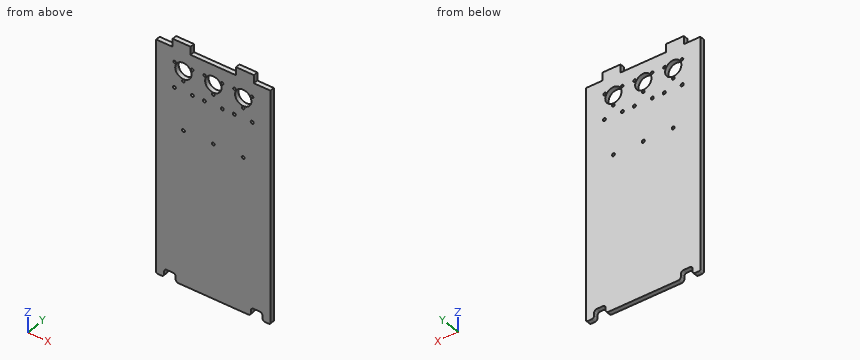
Autodesk Inventor part; units mm, degrees
ref_plane "YZ Plane" through (0, 0, 0) normal (1, 0, 0) x (0, 1, 0)
ref_plane "XZ Plane" through (0, 0, 0) normal (0, 1, 0) x (-1, 0, 0)
ref_plane "XY Plane" through (0, 0, 0) normal (0, 0, 1) x (1, 0, 0)
sketch "Sketch1" plane through (0, 0, 0) normal (0, 1, 0) x (-1, 0, 0)
  line L0 (-41.5, -207.85) -> (-41.5, -204.85)
  line L1 (-44.5, -201.85) -> (-51.2, -201.85)
  line L2 (-54.2, -204.85) -> (-54.2, -207.85)
  line L3 (-57.2, -210.85) -> (-61.5, -210.85)
  arc A0 (-41.5, -207.85) -> (-38.5, -210.85) centre (-38.5, -207.85) ccw
  arc A1 (-41.5, -204.85) -> (-44.5, -201.85) centre (-44.5, -204.85) ccw
  arc A2 (-51.2, -201.85) -> (-54.2, -204.85) centre (-51.2, -204.85) ccw
  arc A3 (-57.2, -210.85) -> (-54.2, -207.85) centre (-57.2, -207.85) ccw
  line L4 (41.5, -207.85) -> (41.5, -204.85)
  line L5 (44.5, -201.85) -> (51.2, -201.85)
  line L6 (54.2, -204.85) -> (54.2, -207.85)
  line L7 (61.5, -210.85) -> (57.2, -210.85)
  line L8 (38.5, -210.85) -> (-38.5, -210.85)
  arc A4 (54.2, -207.85) -> (57.2, -210.85) centre (57.2, -207.85) ccw
  arc A5 (54.2, -204.85) -> (51.2, -201.85) centre (51.2, -204.85) ccw
  arc A6 (44.5, -201.85) -> (41.5, -204.85) centre (44.5, -204.85) ccw
  arc A7 (38.5, -210.85) -> (41.5, -207.85) centre (38.5, -207.85) ccw
  line L9 (44.75, 48.15) -> (25.05, 48.15)
  line L10 (25.05, 48.15) -> (25.05, 57.15)
  line L11 (25.05, 57.15) -> (44.75, 57.15)
  line L12 (44.75, 57.15) -> (44.75, 48.15)
  line L13 (-25.05, 48.15) -> (-44.75, 48.15)
  line L14 (-44.75, 48.15) -> (-44.75, 57.15)
  line L15 (-44.75, 57.15) -> (-25.05, 57.15)
  line L16 (-25.05, 57.15) -> (-25.05, 48.15)
  line L17 (44.75, 48.15) -> (63, 48.15)
  line L18 (25.05, 48.15) -> (-25.05, 48.15)
  line L19 (-44.75, 48.15) -> (-63, 48.15)
  line L20 (63, -209.35) -> (63, 48.15)
  line L21 (-63, -209.35) -> (-63, 48.15)
  arc A8 (61.5, -210.85) -> (63, -209.35) centre (61.5, -209.35) ccw
  arc A9 (-63, -209.35) -> (-61.5, -210.85) centre (-61.5, -209.35) ccw
  point P0 (0, 0)
  point P1 (-47.85, -207.15)
  point P2 (47.85, -207.85)
  point P3 (34.9, 57.15)
  point P4 (-34.9, 57.15)
  point P5 (-59.35, -210.85)
  point P6 (0, -210.85)
  point P7 (59.35, -210.85)
  point P8 (0, 48.15)
  point P9 (-47.85, -201.85)
  point P10 (47.85, -201.85)
  dimension "d3" = 12.7
  dimension "d5" = 3
  dimension "d7" = 12.7
  dimension "d9" = 3
  dimension "d10" = 9
  dimension "d11" = 19.7
  dimension "d13" = 9
  dimension "d14" = 19.7
  dimension "d16" = 1.5
  dimension "d17" = 126
  dimension "d20" = 18.25
  dimension "d21" = 18.25
  dimension "d22" = 57.15
  dimension "d23" = 9
  dimension "d24" = 9
  dimension "d27" = 250
  dimension "d28" = 250
  dimension "d53" = 83
  dimension "d54" = 3.7
extrude "base" add sketch "Sketch1" along normal blind 5
sketch "Sketch2" plane through (0, 5, 0) normal (0, 1, 0) x (1, 0, 0)
  circle A0 centre (0, -26.65) radius 9
  line L0 (-25.05, -48.15) -> (25.05, -48.15)
  line L1 (0, -26.65) -> (-33, -26.65) construction
  point P0 (0, 0)
  dimension "d31" = 18
  dimension "d32" = 21.5
  dimension "d52" = 33
extrude "Poke Hole" cut sketch "Sketch2" against normal up to surface (5 mm away)
pattern_linear "Rectangular Pattern1" count 2 spacing 33 along (-1, 0, 0) count 2 spacing 33 along (1, 0, 0) of "Poke Hole"
sketch "Sketch3" plane through (0, 5, 0) normal (0, 1, 0) x (1, 0, 0)
  circle A0 centre (-33, -15.55) radius 1.5
  circle A1 centre (-33, -26.65) radius 9
  circle A2 centre (-42.6129, -32.2) radius 1.5
  circle A3 centre (-23.3871, -32.2) radius 1.5
  point P0 (0, 0)
  dimension "d41" = 3
  dimension "d42" = 11.1
  dimension "d45" = 360
extrude "Mount Holes" cut sketch "Sketch3" against normal up to surface (5 mm away) contours A0 | A2 | A3
pattern_linear "Rectangular Pattern2" count 3 spacing 33 along (1, 0, 0) of "Mount Holes"
sketch "Sketch4" plane through (0, 5, 0) normal (0, 1, 0) x (1, 0, 0)
  circle A0 centre (-42.875, -4.05) radius 1.65
  circle A1 centre (-23.125, -4.05) radius 1.65
  line L0 (-42.875, -4.05) -> (-23.125, -4.05) construction
  circle A2 centre (-33, -15.55) radius 1.5 construction
  circle A3 centre (-33, 39.3405) radius 1.65
  point P0 (0, 0)
  point P1 (-33, -4.05)
  dimension "d55" = 3.3
  dimension "d56" = 3.3
  dimension "d57" = 19.75
  dimension "d58" = 3.3
  dimension "d59" = 44.5
  dimension "d61" = 11.5
extrude "PCB mount holes" cut sketch "Sketch4" against normal up to surface (5 mm away)
pattern_linear "Rectangular Pattern3" count 3 spacing 33 along (1, 0, 0) of "PCB mount holes"
equation "\"d7\" = d3"
equation "\"d9\" = d5"
equation "\"d10\" = d23"
equation "\"d13\" = d23"
equation "\"d14\" = d11"
equation "\"d21\" = d20"
equation "\"d24\" = d23"
equation "\"d37\" = d52"
equation "\"d40\" = d52"
equation "\"d51\" = d52"
equation "\"d56\" = d55"
equation "\"d58\" = d55"
equation "\"d66\" = d52"
properties part number "front_wall" material "PPS Plastic"
Model file for the job. Use its own axes, mm. Coordinates: 2 decimals unless noted, no trailing zeros. Loops run counter-clockwise (first coordinate to the right, second up) from the corner with the lowest first, then second, coordinate; pieces in that order, holes last. Notation, with made-up numbers: (70, 32) - (122, 32) arc R32 cw to (122, 70) - close; hole circle Ø2 at (33.25, -1.5). An arc over 180 degrees is marked (long way). Answer as a JSON object with one key per item and string values. Group by question number.
(1) Probe line 1 along Z through (x, y) = (0, 2.65); line 2 along X through (y, z) = (3, 15.55); line 3 along X through (y, z) = (4.1, 20). List the from-to ranges inside material, lowest first.
(2) Cut at C-C (y = 2). State how many separate pieces and enclosed holes the cut face has, then the cut area to 3 significant figures.
(3) Flat gauge pins, fed straight in: pin 1 (2.5 mm diameter, centred on y = 1.5, z = 52, fed in from +X); pin 2 (2.5 mm diameter, centred on x = -48, y = 1.5, fed in from -Z). Where does each tip first touch, or does it go through?
(4) Cut at A-A (z = 26.65). Give the cut face in (x, y).
(5) Cut at B-B (x = 5). Give the cut face in (y, z).
Geometry says:
{
 "1": {"line 1": "z = -210.85 to -40.99, -37.69 to 14.05, 17.05 to 17.65, 35.65 to 48.15", "line 2": "x = -63 to -34.5, -31.5 to -1.5, 1.5 to 31.5, 34.5 to 63", "line 3": "x = -63 to -39.06, -26.94 to -6.06, 6.06 to 26.94, 39.06 to 63"},
 "2": {"separate pieces": "1", "enclosed holes": "21", "area": "31,900 mm^2"},
 "3": {"pin 1": "stops at x = 44.75", "pin 2": "stops at z = -201.85"},
 "4": {"outline": "(-63, 0) - (-42, 0) - (-42, 5) - (-63, 5) - close; (-24, 0) - (-9, 0) - (-9, 5) - (-24, 5) - close; (9, 0) - (24, 0) - (24, 5) - (9, 5) - close; (42, 0) - (63, 0) - (63, 5) - (42, 5) - close"},
 "5": {"outline": "(0, -210.85) - (5, -210.85) - (5, 19.17) - (0, 19.17) - close; (0, 34.13) - (5, 34.13) - (5, 48.15) - (0, 48.15) - close"}
}
